Read the model definition and answer for the solid it produces. Units are mm, in the model's axes. Face numbers are marked on the shaded views. A direction names the side the tool comes from. Give positions to 0.01 mm unless a question says otherwise; leave off trailing zeros. Order: outer loops, then holes, each group sorted by start corner. A loop starts at its lowest first (then second) coordinate and runs counter-clockwise, first axis right, second up. Notation, with made-up numbers: M -17.75,32.25 L 35.25,32.25 A26 cw 35.25,50.25 Z; hole C 18.5,-35 d2. An arc over 180 degrees is marked long. One line per item, written item: value.
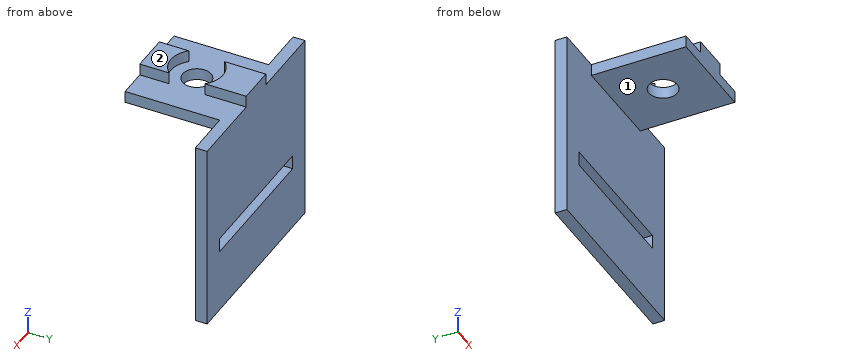
from build123d import *

# Parameters (mm, degrees)
F0_W     = 30
F0_H     = 3
F1_DEPTH = 2.5
F2_DEPTH = 22.5
F0_W_2   = 8
F0_H_2   = 2.5
F3_DEPTH = 22.5
F4_R     = 3
F5_DEPTH = 5.001
F6_START = -2.5
F4_R_2   = 5.5
F6_DEPTH = 2.5


with BuildPart() as f1:
    # F0 (on Front) → F1 (new body)
    with BuildSketch(Plane.XZ):
        Polygon((-20, -20), (20, -20), (20, 17.5), (20, 20), (10, 20), (10, 17.5), (0, 17.5), (-10, 17.5), (-10, 20), (-20, 20), (-20, 17.5), align=None)
        with Locations((0, -5)):
            Rectangle(F0_W, F0_H, mode=Mode.SUBTRACT)
    extrude(amount=F1_DEPTH)

    # F0 (on Front) → F2 (join)
    with BuildSketch(Plane.XZ):
        Polygon((10, 17.5), (10, 20), (4, 20), (-4, 20), (-10, 20), (-10, 17.5), (0, 17.5), align=None)
    extrude(amount=F2_DEPTH)

    # F0 (on Front) → F3 (join)
    with BuildSketch(Plane.XZ):
        with Locations((0, 21.25)):
            Rectangle(F0_W_2, F0_H_2)
    extrude(amount=F3_DEPTH)

    # F4 (on face) → F5 (cut, through all)
    with BuildSketch(Plane(origin=(0, 0, 17.5), x_dir=(1, 0, 0), z_dir=(0, 0, -1))):
        with Locations((0, 12.5)):
            Circle(F4_R)
    extrude(amount=-F5_DEPTH, mode=Mode.SUBTRACT)

    # F4 (on face) → F6 (cut)
    with BuildSketch(Plane(origin=(0, 0, 17.5), x_dir=(1, 0, 0), z_dir=(0, 0, -1)).offset(F6_START)):
        with Locations((0, 12.5)):
            Circle(F4_R_2)
        with Locations((0, 12.5)):
            Circle(F4_R, mode=Mode.SUBTRACT)
    extrude(amount=-F6_DEPTH, mode=Mode.SUBTRACT)


solid = f1.part
1) Find section A-A, the plane x = -8. Write down the section's boundary in (y, z), plus the area to 4 significant figures.
Reported:
outline: M -22.5,17.5 L -2.5,17.5 L -2.5,-3.5 L 0,-3.5 L 0,20 L -22.5,20 Z; M -2.5,-20 L 0,-20 L 0,-6.5 L -2.5,-6.5 Z
area: 142.5 mm^2
2) Find section D-D, the plane x = 0. Write down the section's boundary in (y, z), plus the area to 3 significant figures.
Reported:
outline: M -22.5,17.5 L -15.5,17.5 L -15.5,20 L -18,20 L -18,22.5 L -22.5,22.5 Z; M -9.5,17.5 L -2.5,17.5 L -2.5,-3.5 L 0,-3.5 L 0,22.5 L -7,22.5 L -7,20 L -9.5,20 Z; M -2.5,-20 L 0,-20 L 0,-6.5 L -2.5,-6.5 Z
area: 156 mm^2
3) Each of these flat-tipped pins is pushed along its axis until it touches: pin 1 Ø0.8 at (y, z) = (-3.5, 21.5) entering from +X; pin 2 Ø3.5 at (x, y) = (0, -12.5) entering from +Z; pin 3 Ø2 at (y, z) = (-19.5, 21.5) entering from -X; pin 4 Ø3 at (y, z) = (-15.5, 19) entering from -X. Where does it stop, or does it pass through?
Reported:
pin 1: stops at x = 4
pin 2: passes through
pin 3: stops at x = -4
pin 4: stops at x = -10
4) Find section B-B, the plane y = -12.5. Write down the section's boundary in (x, z), plus the area to 3 significant figures.
Reported:
outline: M -10,17.5 L -3,17.5 L -3,20 L -10,20 Z; M 3,17.5 L 10,17.5 L 10,20 L 3,20 Z
area: 35.0 mm^2
5) Find section C-C, the plane z = 18.5. Write down the section's boundary in (x, y), plus the area to 3 significant figures.
Reported:
outline: M -20,-2.5 L -10,-2.5 L -10,-22.5 L 10,-22.5 L 10,-2.5 L 20,-2.5 L 20,0 L -20,0 Z; hole C 0,-12.5 d6
area: 472 mm^2
6) Consider probe 1 along Z at (x, y) = (-6, -1); probe 2 along X at (y, z) = (-12.5, 19.4); probe 3 along Y at (x, z) = (0, 18.8). Determine where each line is inside the solid, lowest interval first.
Reported:
probe 1: z = -20 to -6.5, -3.5 to 20
probe 2: x = -10 to -3, 3 to 10
probe 3: y = -22.5 to -15.5, -9.5 to 0
7) Which of the six approach directions +Z, -Z, +X, -X, +Y, -Y give full straight-line access (tool end or side, diameter ignored) to the marked faces 1 and 2?
Reported:
face 1: -Z, +X, -X, -Y
face 2: +Z, +X, -X, +Y, -Y
